Geometry check sheet. Reference: the model listing, model coordinates, mm. A direction names the side the tool comes from. Give positions to 0.01 mm unless a question says otherwise; leave off trailing zeros. Loops run counter-clockwise (first coordinate to the right, second up) from the corner with the lowest first, then second, coordinate; pieces in that order, holes last. Notation, with made-up numbers: (-19.75, 15) -> (17.25, 15) arc R26 cw to (17.25, 45) -> close; hole circle Ø3 at (8, 20). An arc over 180 degrees is marked (long way). Answer as a JSON object with one key per item and string values.
from build123d import *

# Parameters (mm, degrees)
SKETCH_1_R      = 1.5
EXTRUDE_1_DEPTH = 5
FILLET_1_R      = 3
SKETCH_2_W      = 14.35
SKETCH_2_H      = 10
SKETCH_2_R      = 1.5
EXTRUDE_2_DEPTH = 10
FILLET_2_R      = 5
FILLET_4_R      = 5.35


with BuildPart() as part:
    # 草图1 → 凸台-拉伸1 (new body)
    with BuildSketch(Plane.XY):
        Polygon((-3, 37.5), (-3, 31.5), (16, 31.5), (16, -11.5), (-3, -11.5), (-3, -17.5), (16, -17.5), (16, -30), (26, -30), (53.26, -30), (53.26, -20), (26, -20), (26, -17.5), (26, 20), (53.26, 20), (53.26, 30), (26, 30), (26, 37.5), align=None)
        with Locations((0, -14.5)):
            Circle(SKETCH_1_R, mode=Mode.SUBTRACT)
        with Locations((0, 34.5)):
            Circle(SKETCH_1_R, mode=Mode.SUBTRACT)
        with Locations((10, 34.5)):
            Circle(SKETCH_1_R, mode=Mode.SUBTRACT)
        with Locations((10, -14.5)):
            Circle(SKETCH_1_R, mode=Mode.SUBTRACT)
    extrude(amount=EXTRUDE_1_DEPTH)

    # 圆角1
    fillet_1_edges = [part.edges().sort_by_distance(p)[0] for p in [
        (26, 20, 2.5),
        (26, -20, 2.5),
        (26, 30, 2.5),
        (26, 37.5, 2.5),
        (16, -30, 2.5),
        (16, -17.5, 2.5),
        (-3, -17.5, 2.5),
        (-3, -11.5, 2.5),
        (-3, 37.5, 2.5),
        (-3, 31.5, 2.5),
    ]]
    fillet(fillet_1_edges, radius=FILLET_1_R - 0.0001)  # a hair under: the kernel refuses the full size

    # 草图2 → 凸台-拉伸2 (add)
    # profile 1 of 2: a face of its own
    with BuildSketch(Plane(origin=(53.26, 0, 0), x_dir=(0, 0, -1), z_dir=(1, 0, 0))):
        with Locations((7.175, 25)):
            Rectangle(SKETCH_2_W, SKETCH_2_H)
        with Locations((9.35, 25)):
            Circle(SKETCH_2_R, mode=Mode.SUBTRACT)
    # profile 2 of 2: a face of its own
    with BuildSketch(Plane(origin=(53.26, 0, 0), x_dir=(0, 0, -1), z_dir=(1, 0, 0))):
        with Locations((7.175, -25)):
            Rectangle(SKETCH_2_W, SKETCH_2_H)
        with Locations((9.35, -25)):
            Circle(SKETCH_2_R, mode=Mode.SUBTRACT)
    extrude(amount=-EXTRUDE_2_DEPTH)

    # 圆角2
    fillet_2_edges = [part.edges().sort_by_distance(p)[0] for p in [
        (48.26, 30, -14.35),
        (48.26, 20, -14.35),
        (48.26, -20, -14.35),
        (48.26, -30, -14.35),
    ]]
    fillet(fillet_2_edges, radius=FILLET_2_R - 0.0001)  # a hair under: the kernel refuses the full size

    # 圆角4
    fillet_4_edges = [part.edges().sort_by_distance(p)[0] for p in [
        (43.26, 25, 0),
        (43.26, -25, 0),
    ]]
    fillet(fillet_4_edges, radius=FILLET_4_R)


solid = part.part
1) Draft check along Z on faces 6 (the face through (48.33, 26.487, -9.155)), 7 (the face through (43.26, -26, -11)), 8 (the face through (48.19, -28.57, -12.85)). Enter one of: pulls with the +Z half, pulls with the -Z half, needs draft (parallel to the pull), parting line crosses it, or undercut.
Geometry check:
{"face 6": "undercut", "face 7": "needs draft", "face 8": "pulls with the -Z half"}
2) Section check B-B on z = -4.5. Record the cut outline in (x, y).
Geometry check:
{"outline": "(43.19, -30) -> (53.26, -30) -> (53.26, -20) -> (43.19, -20) -> close; (43.19, 20) -> (53.26, 20) -> (53.26, 30) -> (43.19, 30) -> close"}
3) Tool access check on faces 1 (the face through (-2.1, -12.36, 2.54)), 2 (the face through (44, 30, 0)), 3 (the face through (48.19, 21.43, -12.85)), 4 (the face through (22, 1, 0)), 5 (the face through (6, -17.5, 2)). Record the directions out of +Z, -Z, +X, -X, +Y, -Y that give a thin tool (end or side, any length) a straight path to the whole face; none if there is none.
Geometry check:
{"face 1": "+Z, -Z, -X", "face 2": "+Z, -Z, +X, +Y", "face 3": "-Z, +X, -X", "face 4": "-Z, -X, +Y, -Y", "face 5": "+Z, -Z, -X, -Y"}
4) Section check D-D on y = -3. Record the cut outline in (x, z).
Geometry check:
{"outline": "(16, 0) -> (26, 0) -> (26, 5) -> (16, 5) -> close"}
5) Section check C-C on x = 10. Record the cut outline in (y, z).
Geometry check:
{"outline": "(-17.5, 0) -> (-16, 0) -> (-16, 5) -> (-17.5, 5) -> close; (-13, 0) -> (-11.5, 0) -> (-11.5, 5) -> (-13, 5) -> close; (31.5, 0) -> (33, 0) -> (33, 5) -> (31.5, 5) -> close; (36, 0) -> (37.5, 0) -> (37.5, 5) -> (36, 5) -> close"}
6) Section check A-A on x = 47. Count the separate pieces of the cut face and the enclosed holes in it, plus the area to 3 significant figures.
Geometry check:
{"separate pieces": "2", "enclosed holes": "2", "area": "351 mm2"}
7) Material ranges on line 1 along Y through (x, z) = (49.5, -9.35); line 2 along Y through (x, z) = (0, 1.15); line 3 along Y through (x, z) = (50.5, -6.5), recorded low to high. Write a range as from..to.
Geometry check:
{"line 1": "y = -30..-26.5, -23.5..-20, 20..23.5, 26.5..30", "line 2": "y = -17.5..-16, -13..-11.5, 31.5..33, 36..37.5", "line 3": "y = -30..-20, 20..30"}
8) Depth check by flat-ended pin: P1, Ø1.5, axis at y = -23, z = 2.5, coming from the -X side; P2, Ø4.5, axis at y = -23, z = -10, coming from the -X side; P3, Ø0.8, axis at y = 33.5, z = 3.5, coming from the +X side; P4, Ø3.5, axis at y = -25, z = -9.35, coming from the +X side. Enter the tip coordinate at first touch or a pass-through.
Geometry check:
{"P1": "stops at x = 16", "P2": "stops at x = 43.26", "P3": "stops at x = 26", "P4": "stops at x = 53.26"}
